from build123d import *

# Parameters (mm, degrees)
SKETCH_1_W               = 64
SKETCH_1_H               = 28
EXTRUDE_1_DEPTH          = 8
SKETCH_2_W               = 54
SKETCH_2_H               = 6
EXTRUDE_2_DEPTH          = 38
FILLET_1_R               = 10
EXTRUDE_3_DEPTH          = 19
EXTRUDE_3_DEPTH_BACK     = 13
CUT_EXTRUDE_1_DEPTH      = 21
CUT_EXTRUDE_1_DEPTH_BACK = 21
SKETCH_5_R               = 4.372337206
SKETCH_5_R_2             = 4
CUT_EXTRUDE_3_DEPTH      = 100


with BuildPart() as part:
    # 草图1 → 凸台-拉伸1 (new body)
    with BuildSketch(Plane(origin=(0, 0, 0), x_dir=(1, 0, 0), z_dir=(0, 1, 0))):
        Rectangle(SKETCH_1_W, SKETCH_1_H)
    extrude(amount=EXTRUDE_1_DEPTH)

    # 草图2 → 凸台-拉伸2 (add)
    with BuildSketch(Plane(origin=(0, 0, 0), x_dir=(1, 0, 0), z_dir=(0, 1, 0))):
        with Locations((0, 11)):
            Rectangle(SKETCH_2_W, SKETCH_2_H)
    extrude(amount=EXTRUDE_2_DEPTH)

    # 圆角1
    fillet_1_edges = [part.edges().sort_by_distance(p)[0] for p in [
        (-27, 38, -11),
        (27, 38, -11),
    ]]
    fillet(fillet_1_edges, radius=FILLET_1_R)

    # 草图3 → 凸台-拉伸3 (add, two sides: drawn at the far end of the back side and taken through both)
    with BuildSketch(Plane.XY.offset(-EXTRUDE_3_DEPTH_BACK)):
        with BuildLine():
            Line((-15, 0), (15, 0))
            ThreePointArc((15, 0), (0, 15), (-15, 0))
        make_face()
    extrude(amount=EXTRUDE_3_DEPTH + EXTRUDE_3_DEPTH_BACK)

    # 草图4 → 切除-拉伸1 (cut, two sides: drawn at the far end of the back side and taken through both)
    with BuildSketch(Plane.XY.offset(-CUT_EXTRUDE_1_DEPTH_BACK)):
        with BuildLine():
            Line((-9, 0), (9, 0))
            ThreePointArc((9, 0), (0, 9), (-9, 0))
        make_face()
    extrude(amount=CUT_EXTRUDE_1_DEPTH + CUT_EXTRUDE_1_DEPTH_BACK, mode=Mode.SUBTRACT)

    # 草图5 → 切除-拉伸3 (cut)
    with BuildSketch(Plane.XY):
        with Locations((-17, 28)):
            Circle(SKETCH_5_R)
        with Locations((17, 28)):
            Circle(SKETCH_5_R_2)
        with BuildLine():
            Line((-8, 28), (-8, 38))
            Line((-8, 38), (8, 38))
            Line((8, 38), (8, 28))
            ThreePointArc((8, 28), (0, 20), (-8, 28))
        make_face()
    extrude(amount=-CUT_EXTRUDE_3_DEPTH, mode=Mode.SUBTRACT)


solid = part.part
Verification items for the finished model (mm, model axes). A direction names the side the tool comes from. Coordinates: 2 decimals unless noted, no trailing zeros. Order: outer loops, then holes, each group sorted by start corner. A loop starts at its lowest first (then second) coordinate and runs counter-clockwise, first axis right, second up. Notation, with made-up numbers: (-14.75, 80.5) -> (14.25, 80.5) arc R21 ccw to (14.25, 119.5) -> close; hole circle Ø4 at (63.5, -30.75). An arc over 180 degrees is marked (long way). Use CSV: the item, a comma, the result in double quotes. Start each with the question number.
Q1. Thickness scan on line 1 along Y through (x, z) = (17, -10.7); line 2 along X through (y, z) = (29.5, -9.5); line 3 along Y through (x, z) = (-17, -12). Record the ranges inside material, lowest first.
Q2. Section check A-A, the plane x = -13.5. Record the cut outline in (y, z).
Q3. Depth check by flat-ended pin: P1, Ø3, axis at y = 35, z = -12, coming from the +X side; P2, Ø6.5, axis at y = 15, z = -10.5, coming from the -X side; P3, Ø1.8, axis at y = 13.5, z = -12, coming from the +X side; P4, Ø5, axis at x = 8.5, z = -6, coming from the +Y side. Enter the tip coordinate at first touch or a pass-through.
Q4. Draft check along X on faces 1 (the cylindrical face through (24.15, 34.99, -11.04)), 2 (the flat face through (8, 33, -11)), 3 (the flat face through (20, 0, 2)). Enter one of: +X half, -X half, draft (parallel to the pull), parting line (faces both ways), or undercut.
Q5. Section check C-C, the plane x = 0. Record the cut outline in (y, z).
Q6. Tool access check on faces 4 (the flat face through (-8, 33, -11)), 5 (the flat face through (-32, 4, 0)), 6 (the flat face through (-27, 18, -11)). Record the directions out of +Z, -Z, +X, -X, +Y, -Y that give a thin tool (end or side, any length) a straight path to the whole face; none if there is none.
Q7. Section check B-B, the plane z = -3.5. Record the cut outline in (x, y).
Q8. Section check D-D, the plane x = 12. Record the cut outline in (y, z).
Returned:
1,line 1,"y = 0 to 24, 32 to 38"
1,line 2,"x = -26.89 to -21.11, -12.89 to -8, 8 to 13.29, 20.71 to 26.89"
1,line 3,"y = 0 to 23.63, 32.37 to 38"
2,outline,"(0, -14) -> (25.38, -14) -> (25.38, -8) -> (8, -8) -> (8, 14) -> (6.54, 14) -> (6.54, 19) -> (0, 19) -> close; (30.62, -14) -> (38, -14) -> (38, -8) -> (30.62, -8) -> close"
3,P1,"stops at x = 25.35"
3,P2,"stops at x = -27"
3,P3,"stops at x = 27"
3,P4,"stops at y = 38"
4,face 1,"+X half"
4,face 2,"undercut"
4,face 3,"draft"
5,outline,"(9, -14) -> (20, -14) -> (20, -8) -> (15, -8) -> (15, 19) -> (9, 19) -> close"
6,face 4,"+Z, -Z, +Y"
6,face 5,"+Z, -Z, -X, +Y, -Y"
6,face 6,"+Z, -Z, -X, +Y"
7,outline,"(-32, 0) -> (-9, 0) arc R9 cw to (9, 0) -> (32, 0) -> (32, 8) -> (12.69, 8) arc R15 ccw to (-12.69, 8) -> (-32, 8) -> close"
8,outline,"(0, -14) -> (38, -14) -> (38, -8) -> (9, -8) -> (9, 19) -> (0, 19) -> close"
